from build123d import *

# Parameters (mm, degrees)
CHAMFER_1_SIZE  = 0.2
SKETCH_4_R      = 0.45
SKETCH_5_R      = 0.3
EXTRUDE_2_DEPTH = 15


# Read off the part's stored shape, not the designer's step: 旋转2
with BuildPart() as part:
    # 旋转2 outline → 旋转2 (revolve)
    with BuildSketch(Plane.YX):
        Polygon((3.1, 0), (0, 0), (0, -27), (2, -27), (2.75, -20), (2.9, -10), (3.1, -10), align=None)
    revolve(axis=Axis((0, 0, 0), (1, 0, 0)))

    # 倒角1
    chamfer_1_edges = [part.edges().sort_by_distance(p)[0] for p in [
        (-10, -3.1, 0),
    ]]
    chamfer(chamfer_1_edges, length=CHAMFER_1_SIZE - 0.0001)  # a hair under: the kernel refuses the full size

    # 扫描1: sweep along a path in 草图3
    with BuildLine(Plane.XY) as sweep_1_path:
        ThreePointArc((-27, 0), (-30.535533906, -1.464466094), (-32, -5))
    # 草图4 → 扫描1 (sweep)
    with BuildSketch(Plane.ZY.offset(27)):
        Circle(SKETCH_4_R)
    sweep(path=sweep_1_path.line)

    # 草图5 → 拉伸2 (add)
    with BuildSketch(Plane(origin=(0, 0, 0), x_dir=(0, 0, -1), z_dir=(1, 0, 0))):
        with Locations(Location((-0.635, 0.635, 0), (0, 0, 270))):
            Circle(SKETCH_5_R)
        with Locations(Location((-0.635, -0.635, 0), (0, 0, 270))):
            Circle(SKETCH_5_R)
        with Locations(Location((0.635, 0.635, 0), (0, 0, 270))):
            Circle(SKETCH_5_R)
        with Locations(Location((0.635, -0.635, 0), (0, 0, 270))):
            Circle(SKETCH_5_R)
    extrude(amount=EXTRUDE_2_DEPTH)


solid = part.part
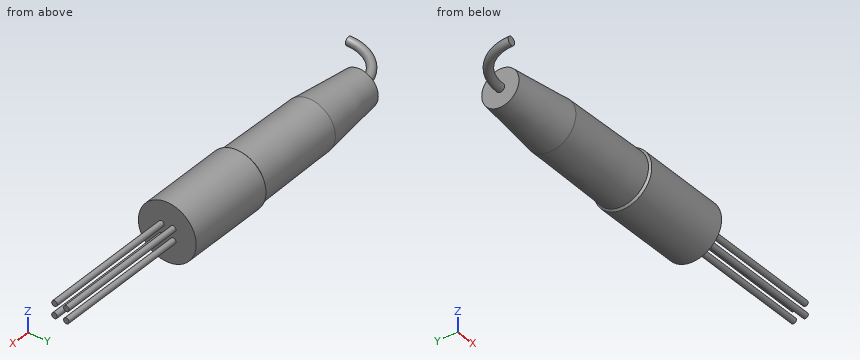
Here's how the part is built. I have some questions about the finished solid (model axes, mm). Coordinates: 2 decimals unless noted, no trailing zeros. Write each loop counter-clockwise with the first axis right and the second up, starting at its lowest first coordinate (ties: lowest second). Pieces come first, ordered by that corner, then holes.
Item 1: I want a section at A-A on x = -8.5. Write out the boundary of the cut face in (y, z), and give its area (3 significant figures).
Item 2: I want a section at B-B on x = 12. Write out the boundary of the cut face in (y, z) (3 decimals), and give its area (3 significant figures).
Item 3: If I drill on line 1 (Y direction, x = 5, z = -0.5); line 2 (Z direction, x = -29.5, y = -0.75); line 3 (Z direction, x = -20.5, y = -1.25), over which ranges is the centre line in solid material (lowest first)?
Item 4: Will these pins go through, and if not, where does the flat tip stop? pin 1 (1.5 mm diameter, centred on y = 0.5, z = -2.5, fed in from +X); pin 2 (1.5 mm diameter, centred on y = 1, z = 2.5, fed in from -X); pin 3 (3 mm diameter, centred on y = 0.5, z = -0.5, fed in from -X).
Findings below:
1. outline: circle Ø6.2 at (0, 0)
1. area: 30.2 mm2
2. outline: circle Ø0.6 at (-0.635, -0.635); circle Ø0.6 at (-0.635, 0.635); circle Ø0.6 at (0.635, -0.635); circle Ø0.6 at (0.635, 0.635)
2. area: 1.13 mm2
3. line 1: y = -0.9 to -0.37, 0.37 to 0.9
3. line 2: z = -0.44 to 0.44
3. line 3: z = -2.39 to 2.39
4. pin 1: stops at x = 0
4. pin 2: stops at x = -27
4. pin 3: stops at x = -30.63
